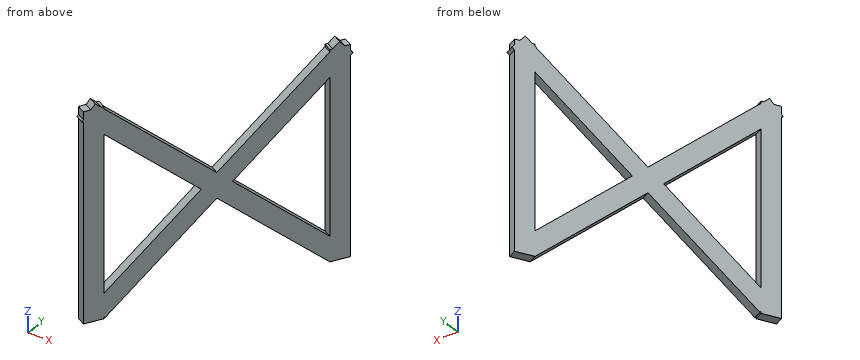
from build123d import *

# Parameters (mm, degrees)
BOX220_W                  = 0.5
BOX220_H                  = 1
BOX220_DEPTH              = 11
BOX221_W                  = 0.5
BOX221_H                  = 1
BOX221_DEPTH              = 16
BOX221_ROLL_ANGLE         = 49
BOX222_W                  = 0.5
BOX222_H                  = 1
BOX222_DEPTH              = 16
BOX222_ROLL_ANGLE         = -49
BOX219_W                  = 0.5
BOX219_H                  = 1
BOX219_DEPTH              = 11
FUSION017_PLACEMENT_ANGLE = 30


with BuildPart() as cubo220:
    # Box220 → Box220 (new body)
    with BuildSketch(Plane(origin=(0, 12, 0.5), x_dir=(1, 0, 0), z_dir=(0, 0, 1))):
        with Locations((0.25, 0.5)):
            Rectangle(BOX220_W, BOX220_H)
    extrude(amount=BOX220_DEPTH)


with BuildPart() as cubo221:
    # Box221 → Box221 (new body)
    with BuildSketch(Plane.XY):
        with Locations((0.25, 0.5)):
            Rectangle(BOX221_W, BOX221_H)
    extrude(amount=BOX221_DEPTH)


with BuildPart() as cubo221_1:
    # Box221 roll: moved
    add(cubo221.part.rotate(Axis((0, 0, 0), (1, 0, 0)), BOX221_ROLL_ANGLE))


with BuildPart() as cubo221_2:
    # Box221 placement: moved
    add(cubo221_1.part.moved(Location((0, 12, 0.5))))


with BuildPart() as cubo222:
    # Box222 → Box222 (new body)
    with BuildSketch(Plane.XY):
        with Locations((0.25, 0.5)):
            Rectangle(BOX222_W, BOX222_H)
    extrude(amount=BOX222_DEPTH)


with BuildPart() as cubo222_1:
    # Box222 roll: moved
    add(cubo222.part.rotate(Axis((0, 0, 0), (1, 0, 0)), BOX222_ROLL_ANGLE))


with BuildPart() as cubo222_2:
    # Box222 placement: moved
    add(cubo222_1.part.moved(Location((0, 0.4, 1.3))))


with BuildPart() as fusion017:
    # Box219 → Box219 (new body)
    with BuildSketch(Plane.XY.offset(0.5)):
        with Locations((0.25, 0.5)):
            Rectangle(BOX219_W, BOX219_H)
    extrude(amount=BOX219_DEPTH)

    # Fusion017: union Cubo220, Cubo221, Cubo222
    add(cubo220.part)
    add(cubo221_2.part)
    add(cubo222_2.part)


with BuildPart() as fusion017_1:
    # Fusion017 placement: moved
    add(fusion017.part.moved(Location((-210.5, 102.8, 0))).rotate(Axis((-210.5, 102.8, 0), (0, 0, -1)), FUSION017_PLACEMENT_ANGLE))


solid = fusion017_1.part
Model file for the job. Use its own axes, mm. Round coordinates to 2 decimals unless told otherwise and drop trailing zeros. Loops run counter-clockwise (first coordinate to the right, second up) from the corner with the lowest first, then second, coordinate; pieces in that order, holes last.
1. Band-saw the part on A-A, the plane z = 4. List the corners of the cut face in (x, y), and give its area (3 significant figures).
Check values:
outline: (-210.5, 102.8) - (-210.07, 102.55) - (-209.57, 103.42) - (-210, 103.67) - close; (-208.75, 105.84) - (-208.31, 105.59) - (-207.55, 106.91) - (-207.98, 107.16) - close; (-206.51, 109.71) - (-206.08, 109.46) - (-205.32, 110.78) - (-205.75, 111.03) - close; (-204.5, 113.19) - (-204.07, 112.94) - (-203.57, 113.81) - (-204, 114.06) - close
area: 2.52 mm2
2. Wall check: probe 1 along Z at (x, y) = (-209.75, 103.75); probe 2 along Z at (x, y) = (-207.75, 107); probe 3 along X at (y, z) = (107.25, 7.25). Give the ranges that are in metal, low to high.
Check values:
probe 1: z = 0.67 to 1.99, 9.89 to 11.22
probe 2: z = 3.98 to 5.31, 6.57 to 7.9
probe 3: x = -207.93 to -207.35
3. Drop flat-ended pins along their axis: P1, Ø5, axis at y = 105.5, z = 5, coming from the +X side; P2, Ø3, axis at y = 107.5, z = 8, coming from the -X side; P3, Ø4, axis at x = -206.5, y = 106, coming from the +Z side. Give the stop position or say it passes through.
Check values:
P1: stops at x = -206.92
P2: stops at x = -208.65
P3: stops at z = 9.38
4. Band-saw the part on C-C, the plane y = 110.25. List the corners of the cut face in (x, z).
Check values:
outline: (-206.2, 3.45) - (-205.62, 3.2) - (-205.62, 4.53) - (-206.2, 4.78) - close; (-206.2, 7.11) - (-205.62, 7.36) - (-205.62, 8.68) - (-206.2, 8.43) - close
5. Band-saw the part on B-B, the plane x = -205. List the corners of the cut face in (y, z), and give its area (3 significant figures).
Check values:
outline: (111.33, 2.12) - (112.33, 1.37) - (112.33, 2.69) - (111.33, 3.45) - close; (111.33, 8.44) - (112.33, 9.19) - (112.33, 10.51) - (111.33, 9.76) - close
area: 2.65 mm2
